The drawing under review shows one solid part. Ordinate dimensions are in mm from its lowest x, y, z. A direction names the side the tool comes from. Give positions to 0.01 mm unless a question says otherwise; leave off trailing zeros. Order: outer loops, then holes, each group sorted by start corner. A loop starts at its lowest first (then second) coordinate and runs counter-clockwise, first axis right, second up. Notation, with made-up numbers: (24.5, -29.5) -> (33.5, -29.5) arc R22 cw to (33.5, -14.5) -> close; hole circle Ø4 at (12, 18). An arc over 180 degrees is marked (long way). One line per item, written item: value.
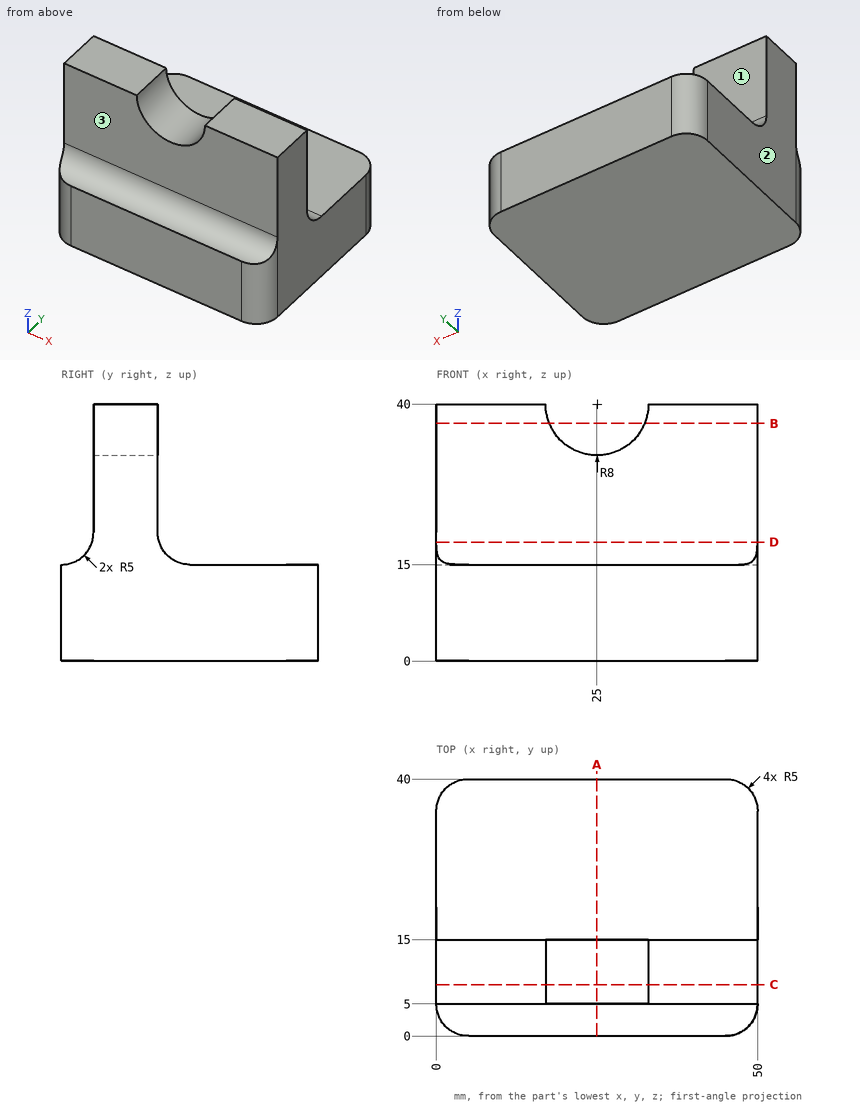
Item 1: Add section C-C on y = 8. Give the boundary of the cut face in (x, z).
Returned:
outline: (0, 0) -> (50, 0) -> (50, 40) -> (33, 40) arc R8 cw to (17, 40) -> (0, 40) -> close
Item 2: Add section D-D on z = 18.5. Give the boundary of the cut face in (x, y), plus the area to 3 significant figures.
Returned:
outline: (0, 5) arc R5 ccw to (0.01, 4.77) -> (49.99, 4.77) arc R5 ccw to (50, 5) -> (50, 15.23) -> (0, 15.23) -> close
area: 523 mm²
Item 3: Add section A-A on x = 25. Give the boundary of the cut face in (y, z), plus the area to 3 significant figures.
Returned:
outline: (0, 0) -> (40, 0) -> (40, 15) -> (20, 15) arc R5 cw to (15, 20) -> (15, 32) -> (5, 32) -> (5, 20) arc R5 cw to (0, 15) -> close
area: 781 mm²
Item 4: Add section B-B on z = 37. Give the boundary of the cut face in (x, y).
Returned:
outline: (0, 5) -> (17.58, 5) -> (17.58, 15) -> (0, 15) -> close; (32.42, 5) -> (50, 5) -> (50, 15) -> (32.42, 15) -> close
Item 5: Clearance check with flat-ended pins moving along their axes: P1, Ø10, axis at x = 18, z = 26.5, coming from the +Y side; P2, Ø1, axis at x = 41.5, z = 19, coming from the -Y side; P3, Ø12, axis at x = 42, z = 25, coming from the -Y side. State where each tip first meets the part, or that it passes through.
Returned:
P1: y = 15
P2: y = 4.77
P3: y = 4.9
Item 6: To check wall thickness, follow line 1 along Z through (x, y) = (43, 37); line 2 along Z through (x, y) = (31.5, 4); line 3 along Y through (x, z) = (31, 23). State the ranges of each line that lie inside material, in increasing order. Write a range as from..to.
Returned:
line 1: 0..15
line 2: 0..17
line 3: 5..15
Item 7: Machinability: for the marked faces 1, 2 and 3, which of the approach directions +Z, -Z, +X, -X, +Y, -Y give a long, thin tool a straight path to every point of the face, cutting with its end or side? Answer none if there is none.
Returned:
face 1: +Z, +X, -X, +Y
face 2: +Z, -Z, -X, +Y, -Y
face 3: +Z, +X, -X, -Y
